The drawing under review shows one solid part. Ordinate dimensions are in mm from its lowest x, y, z. A direction names the side the tool comes from. Coordinates: 2 decimals unless noted, no trailing zeros. Loops run counter-clockwise (first coordinate to the right, second up) from the corner with the lowest first, then second, coordinate; pieces in that order, holes last.
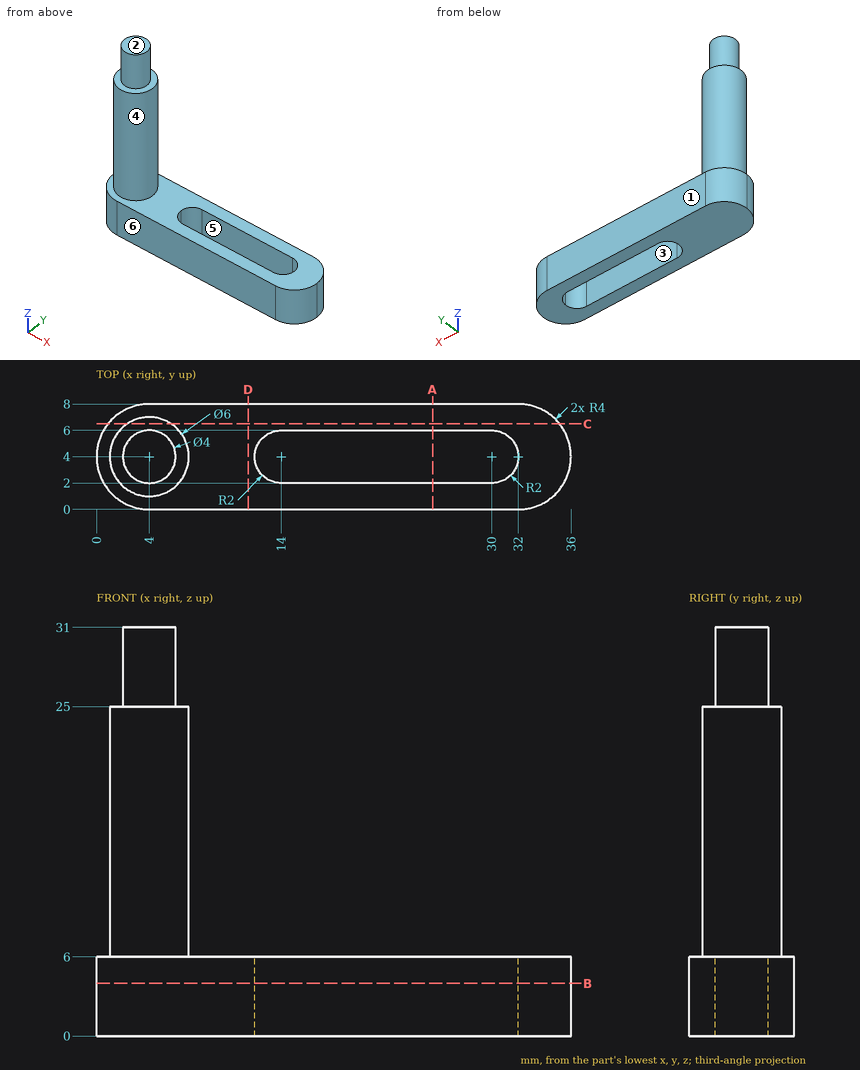
Q1. Machinability: for the marked faces 4, 5 and 6, which of the approach directions +Z, -Z, +X, -X, +Y, -Y give a long, thin tool a straight path to every point of the face, cutting with its end or side? Answer none if there is none.
Q2. Clearance check with flat-ended pins moving along their axes: pin 1 Ø4 at (y, z) = (3.5, 22.5) entering from +X; pin 2 Ø3 at (x, y) = (15, 1) entering from +Z. State where each tip first meets the part, or that it passes through.
Q3. The part is to be moulded in two halves that separate along Y. For the marked faces 1, 2 and 3, say which applies: pulls with the +Y half, pulls with the -Y half, needs draft (parallel to the pull), parting line crosses it, or undercut.
Q4. Take a section at A-A, the plane x = 25.5. Write out the cut boundary in (y, z), then the cut area to 3 significant figures.
Q5. Take a section at D-D, the plane x = 11.5. Write out the cut boundary in (y, z), then the cut area to 3 significant figures.
Q6. For line 1 (Y direction, x = 23, z = 3); line 2 (Z direction, x = 26, y = 7.25); line 3 (X direction, y = 6.75, z = 9), list the stretches that pass through material, from the lowest coordinate up.
Q7. Take a section at C-C, the plane y = 6.5. Write out the cut boundary in (x, z).
Q8. Take a section at B-B, the plane z = 4. Write out the cut boundary in (x, y).
Entries:
1. face 4: +Z
1. face 5: +Z, -Z
1. face 6: +Z, -Z, +X, -X, -Y
2. pin 1: stops at x = 7
2. pin 2: stops at z = 6
3. face 1: pulls with the +Y half
3. face 2: needs draft
3. face 3: undercut
4. outline: (0, 0) - (2, 0) - (2, 6) - (0, 6) - close; (6, 0) - (8, 0) - (8, 6) - (6, 6) - close
4. area: 24.0 mm2
5. outline: (0, 0) - (8, 0) - (8, 6) - (0, 6) - close
5. area: 48.0 mm2
6. line 1: y = 0 to 2, 6 to 8
6. line 2: z = 0 to 6
6. line 3: x = 2.8 to 5.2
7. outline: (0.88, 0) - (35.12, 0) - (35.12, 6) - (5.66, 6) - (5.66, 25) - (2.34, 25) - (2.34, 6) - (0.88, 6) - close
8. outline: (4, 0) - (32, 0) arc R4 ccw to (32, 8) - (4, 8) arc R4 ccw to start; hole (12, 4) arc R2 ccw to (14, 2) - (30, 2) arc R2 ccw to (32, 4) arc R2 ccw to (30, 6) - (14, 6) arc R2 ccw to start
